from build123d import *

# Parameters (mm, degrees)
SKETCH_1_W          = 250
SKETCH_1_H          = 300
EXTRUDE_1_DEPTH     = 300
SKETCH_2_W          = 230
SKETCH_2_H          = 280
CUT_EXTRUDE_1_DEPTH = 290
SKETCH_3_W          = 295
SKETCH_3_H          = 360
EXTRUDE_2_DEPTH     = 10
CUT_EXTRUDE_2_DEPTH = 10


with BuildPart() as part:
    # 草图1 → 凸台-拉伸1 (new body)
    with BuildSketch(Plane.XY):
        with Locations((125, 150)):
            Rectangle(SKETCH_1_W, SKETCH_1_H)
    extrude(amount=EXTRUDE_1_DEPTH)

    # 草图2 → 切除-拉伸1 (cut)
    with BuildSketch(Plane.XY.offset(300)):
        with Locations((125, 150)):
            Rectangle(SKETCH_2_W, SKETCH_2_H)
    extrude(amount=-CUT_EXTRUDE_1_DEPTH, mode=Mode.SUBTRACT)

    # 草图3 → 凸台-拉伸2 (add)
    with BuildSketch(Plane.XZ):
        with Locations((132.5, 150)):
            Rectangle(SKETCH_3_W, SKETCH_3_H)
    extrude(amount=EXTRUDE_2_DEPTH)

    # 草图4 → 切除-拉伸2 (cut)
    with BuildSketch(Plane(origin=(0, -10, 0), x_dir=(-1, 0, 0), z_dir=(0, -1, 0))):
        with BuildLine():
            Line((-101.811483313, -287.738071641), (-183.649909723, -287.738071641))
            ThreePointArc((-183.649909723, -287.738071641), (-201.387981364, -270), (-183.649909723, -252.261928359))
            Line((-183.649909723, -252.261928359), (-101.811483313, -252.261928359))
            ThreePointArc((-101.811483313, -252.261928359), (-84.073411671, -270), (-101.811483313, -287.738071641))
        make_face()
    extrude(amount=-CUT_EXTRUDE_2_DEPTH, mode=Mode.SUBTRACT)


solid = part.part
Read the model definition and answer for the solid it produces. Units are mm, in the model's axes. A direction names the side the tool comes from. Give positions to 0.01 mm unless a question says otherwise; leave off trailing zeros. Loops run counter-clockwise (first coordinate to the right, second up) from the corner with the lowest first, then second, coordinate; pieces in that order, holes last. Notation, with made-up numbers: (-4.5, -4.75) -> (49.5, -4.75) arc R15 cw to (49.5, 20.25) -> close; hole circle Ø11 at (79, -21.5). An arc over 180 degrees is marked (long way). Answer as CSV lines item,"result".
Item 1: Determine the mould class of faces 1 (the face through (84.078, -5.07, 269.61)), 2 (the face through (130, -5, -30)), 3 (the face through (123, 152, 10)), 4 (the face through (130, -10, 153)) for opening direction Z: +Z half, -Z half, draft (parallel to the pull), parting line (faces both ways), or undercut.
Returned:
face 1,"undercut"
face 2,"-Z half"
face 3,"+Z half"
face 4,"draft"
Item 2: Find section A-A on z = 89.5. Give the vertices of the cut face in (x, y).
Returned:
outline,"(-15, -10) -> (280, -10) -> (280, 0) -> (250, 0) -> (250, 300) -> (0, 300) -> (0, 0) -> (-15, 0) -> close; hole (10, 10) -> (240, 10) -> (240, 290) -> (10, 290) -> close"
Item 3: Find section D-D on z = 270. Give the vertices of the cut face in (x, y), plus the area to 3 significant figures.
Returned:
outline,"(-15, -10) -> (84.07, -10) -> (84.07, 0) -> (201.39, 0) -> (201.39, -10) -> (280, -10) -> (280, 0) -> (250, 0) -> (250, 300) -> (0, 300) -> (0, 0) -> (-15, 0) -> close; hole (10, 10) -> (240, 10) -> (240, 290) -> (10, 290) -> close"
area,"12,400 mm²"
Item 4: For faces 5 (the face through (4, 151, 300)), 6 (the face through (143, -5, 252.262)), 7 (the face through (123, 10, 157)), 8 (the face through (0, 148, 148)), determine the directions among +Z, -Z, +X, -X, +Y, -Y from which every point of the face is accessible in a straight line to the end or side of a thin tool.
Returned:
face 5,"+Z, +X, -X, +Y"
face 6,"-Y"
face 7,"+Z"
face 8,"+Z, -Z, -X, +Y"
Item 5: Find section C-C on y = 177. Give the vertices of the cut face in (x, z), plus the area to 3 significant figures.
Returned:
outline,"(0, 0) -> (250, 0) -> (250, 300) -> (240, 300) -> (240, 10) -> (10, 10) -> (10, 300) -> (0, 300) -> close"
area,"8,300 mm²"
Item 6: Consider line 1 (X direction, y = 87, z = 235); line 2 (Y direction, x = 62.5, z = 18.5); line 3 (Z direction, x = 74.5, y = 246.5). Determine where each line is inside the solid, lowest interval first. Write a range as [from, to].
Returned:
line 1,"x = [0, 10], [240, 250]"
line 2,"y = [-10, 10], [290, 300]"
line 3,"z = [0, 10]"
Item 7: Find section B-B on x = 42. Give the vertices of the cut face in (y, z), plus the area to 3 significant figures.
Returned:
outline,"(-10, -30) -> (0, -30) -> (0, 0) -> (300, 0) -> (300, 300) -> (290, 300) -> (290, 10) -> (10, 10) -> (10, 300) -> (0, 300) -> (0, 330) -> (-10, 330) -> close"
area,"12,400 mm²"
Item 8: Each of these flat-tipped pins is pushed along its axis until it touches: pin 1 (12 mm diameter, centred on x = 42.5, y = 233, fed in from -Z); pin 2 (3 mm diameter, centred on y = 140.5, z = 263.5, fed in from -X). Where does it stop, or does it pass through?
Returned:
pin 1,"stops at z = 0"
pin 2,"stops at x = 0"
